from build123d import *

# Parameters (mm, degrees)
SKETCH_1_R          = 1.5
SKETCH_1_R_2        = 7
EXTRUDE_1_DEPTH     = 2.25
SKETCH_3_W          = 19.5
SKETCH_3_H          = 40
EXTRUDE_2_DEPTH     = 3
SKETCH_4_R          = 1.5
CUT_EXTRUDE_1_DEPTH = 227.967348396
SKETCH_5_W          = 4.5
SKETCH_5_H          = 15.072529032
EXTRUDE_3_DEPTH     = 20
CUT_EXTRUDE_3_DEPTH = 10


with BuildPart() as part:
    # 草图1 → 凸台-拉伸1 (new, symmetric)
    with BuildSketch(Plane(origin=(0, 0, 0), x_dir=(0, 0, -1), z_dir=(1, 0, 0))):
        with BuildLine():
            ThreePointArc((102.736907967, -10), (110.379173808, -11.526455333), (116.85785315, -15.85785315))
            Line((116.85785315, -15.85785315), (171, -70))
            Line((171, -70), (199.284271247, -70))
            Line((199.284271247, -70), (125.142135624, 4.142135624))
            ThreePointArc((125.142135624, 4.142135624), (118.653668647, 8.47759065), (111, 10))
            Line((111, 10), (16, 10))
            ThreePointArc((16, 10), (11.149287499, 10.597149997), (6.588235294, 12.352941176))
            ThreePointArc((6.588235294, 12.352941176), (3.395498751, 13.581995002), (0, 14))
            Line((0, 14), (-18, 14))
            Line((-18, 14), (-18, 11))
            Line((-18, 11), (-13.388941598, -4.090995342))
            ThreePointArc((-13.388941598, -4.090995342), (-8.328447191, -11.253309175), (0, -14))
            Line((0, -14), (13.224243357, -14))
            Line((13.224243357, -14), (13.224243357, -10.193557234))
            ThreePointArc((13.224243357, -10.193557234), (14.608751519, -10.048447989), (16, -10))
            Line((16, -10), (102.736907967, -10))
        make_face()
        with Locations((164.036406871, -48.894271247)):
            Circle(SKETCH_1_R, mode=Mode.SUBTRACT)
        with Locations((142.823203436, -27.681067812)):
            Circle(SKETCH_1_R, mode=Mode.SUBTRACT)
        with Locations((0, -10.5)):
            Circle(SKETCH_1_R, mode=Mode.SUBTRACT)
        with Locations((-10.5, 0)):
            Circle(SKETCH_1_R, mode=Mode.SUBTRACT)
        Circle(SKETCH_1_R_2, mode=Mode.SUBTRACT)
        with Locations((10.5, 0)):
            Circle(SKETCH_1_R, mode=Mode.SUBTRACT)
        with Locations((0, 10.5)):
            Circle(SKETCH_1_R, mode=Mode.SUBTRACT)
        with Locations((40.5, 0)):
            Circle(SKETCH_1_R, mode=Mode.SUBTRACT)
        with Locations((70.5, 0)):
            Circle(SKETCH_1_R, mode=Mode.SUBTRACT)
        with Locations((121.61, -6.467864376)):
            Circle(SKETCH_1_R, mode=Mode.SUBTRACT)
        with Locations((100.5, 0)):
            Circle(SKETCH_1_R, mode=Mode.SUBTRACT)
    extrude(amount=EXTRUDE_1_DEPTH, both=True)

    # 草图3 → 凸台-拉伸2 (add)
    with BuildSketch(Plane.XZ.offset(70)):
        with Locations((-7.5, -190.144271247)):
            Rectangle(SKETCH_3_W, SKETCH_3_H)
    extrude(amount=EXTRUDE_2_DEPTH)

    # 草图4 → 切除-拉伸1 (cut, through all)
    with BuildSketch(Plane(origin=(0, -70, 0), x_dir=(1, 0, 0), z_dir=(0, 1, 0))):
        with Locations(Location((-10.25, 203.144271247, 0), (0, 0, 270))):
            Circle(SKETCH_4_R)
        with Locations(Location((-10.25, 177.144271247, 0), (0, 0, 90))):
            Circle(SKETCH_4_R)
    extrude(amount=-CUT_EXTRUDE_1_DEPTH, mode=Mode.SUBTRACT)

    # 草图5 → 凸台-拉伸3 (add)
    with BuildSketch(Plane(origin=(0, 64.642135624, -64.642135624), x_dir=(1, 0, 0), z_dir=(0, 0.7071067811865465, -0.7071067811865487))):
        with Locations((0, 162.87646975)):
            Rectangle(SKETCH_5_W, SKETCH_5_H)
    extrude(amount=EXTRUDE_3_DEPTH)

    # 草图9 → 切除-拉伸3 (cut)
    with BuildSketch(Plane.ZY.offset(2.25)):
        Polygon((-196.699542099, -39.130999604), (-174.484248136, -45.199976888), (-188.626383759, -31.057841264), align=None)
    extrude(amount=-CUT_EXTRUDE_3_DEPTH, mode=Mode.SUBTRACT)


solid = part.part
Read the model definition and answer for the solid it produces. Units are mm, in the model's axes. A direction names the side the tool comes from. Coordinates: 2 decimals unless noted, no trailing zeros. Write each loop counter-clockwise with the first axis right and the second up, starting at its lowest first coordinate (ties: lowest second). Pieces come first, ordered by that corner, then holes. Notation, with made-up numbers: M 42.25,56 L 87.25,56 A12 cw 87.25,70 Z; hole C 8,50 d11. An arc over 180 degrees is marked long. Use a Markdown table: item, result.
Q1. Straight lines are drawn through the part: L1, parallel to Y at x = 0.65, z = 0; L2, parallel to X at y = 1, z = -19; L3, parallel to Y at x = -1, z = -63. For each, find the intervals that lie inside material, in ascending order. Write a range as [from, to].
Answer block:
| item | result |
|---|---|
| L1 | y = [-14, -12], [-9, -7], [7, 9], [12, 14] |
| L2 | x = [-2.25, 2.25] |
| L3 | y = [-10, 10] |
Q2. The part is cut by section B-B, the plane z = -75. Write down the section's boundary in (x, y), then the cut area to 3 significant figures.
Answer block:
| item | result |
|---|---|
| outline | M -2.25,-10 L 2.25,-10 L 2.25,10 L -2.25,10 Z |
| area | 90.0 mm2 |
Q3. The part is cut by section C-C, the plane y = -37. Write down the section's boundary in (x, z), then the cut area to 3 significant figures.
Answer block:
| item | result |
|---|---|
| outline | M -2.25,-166.28 L 2.25,-166.28 L 2.25,-138 L -2.25,-138 Z |
| area | 127 mm2 |
Q4. Which of the six approach directions +Z, -Z, +X, -X, +Y, -Y give full straight-line access (tool end or side, diameter ignored) to faces 4 (the face through (0.031, -11.485, -110.278)), 5 (the face through (0, -49, -192)), 6 (the face through (-2.25, -6, -98))?
Answer block:
| item | result |
|---|---|
| face 4 | +X, -X, -Y |
| face 5 | -Z, +X, -X |
| face 6 | +Z, -Z, -X, +Y |
Q5. Each of these flat-tipped pins is pushed along its axis until it touches: pin 1 Ø8 at (x, y) = (-3, -15) entering from +Z; pin 2 Ø1.3 at (x, z) = (-1, -40) entering from +Y; pin 3 Ø4 at (y, z) = (0, -70.5) entering from -X. Where does it stop, or does it pass through?
Answer block:
| item | result |
|---|---|
| pin 1 | stops at z = 8.57 |
| pin 2 | stops at y = 10 |
| pin 3 | stops at x = -2.25 |
Q6. The part is cut by section A-A, the plane z = -191. Write down the section's boundary in (x, y).
Answer block:
| item | result |
|---|---|
| outline | M -17.25,-73 L 2.25,-73 L 2.25,-61.72 L -2.25,-61.72 L -2.25,-70 L -17.25,-70 Z; M -2.25,-50 L 2.25,-50 L 2.25,-40.69 L -2.25,-40.69 Z |
Q7. Determine the mould class of faces 1 (the face through (0.031, -63.028, -192.312)), 2 (the face through (-8, -73, -190)), 3 (the face through (0, -12, -13.224)) for opening direction Z: released by +Z, released by -Z, zero draft, split by the parting line, or undercut.
Answer block:
| item | result |
|---|---|
| face 1 | released by -Z |
| face 2 | zero draft |
| face 3 | undercut |
